```python
from build123d import *

# Parameters (mm, degrees)
SKETCH3_W           = 0.5
SKETCH3_H           = 0.5
BOSS_EXTRUDE1_DEPTH = 10
SKETCH4_W           = 0.5
SKETCH4_H           = 0.5
BOSS_EXTRUDE2_DEPTH = 5
SKETCH5_R           = 0.5
BOSS_EXTRUDE3_DEPTH = 5


with BuildPart() as part:
    # Sketch2 → Revolve1 (revolve)
    with BuildSketch(Plane.XY, mode=Mode.PRIVATE) as revolve1_sk:
        Polygon((0, 0), (2.48, 0), (2.37, 7.9), (0, 7.9), align=None)
    revolve(revolve1_sk.sketch.rotate(Axis((0, 7.9, 0), (0, -1, 0)), 180), axis=Axis((0, 7.9, 0), (0, -1, 0)))

    # Sketch3 → Boss-Extrude1 (add)
    with BuildSketch(Plane.XZ):
        with Locations((-0.625, 0)):
            Rectangle(SKETCH3_W, SKETCH3_H)
        with Locations((-1.875, 0)):
            Rectangle(SKETCH3_W, SKETCH3_H)
        with Locations((0.625, 0)):
            Rectangle(SKETCH3_W, SKETCH3_H)
        with Locations((1.875, 0)):
            Rectangle(SKETCH3_W, SKETCH3_H)
    extrude(amount=BOSS_EXTRUDE1_DEPTH)

    # Sketch4 → Boss-Extrude2 (add)
    with BuildSketch(Plane.XY.offset(-0.25)):
        with Locations((-1.875, -9.75)):
            Rectangle(SKETCH4_W, SKETCH4_H)
        with Locations((-0.625, -9.75)):
            Rectangle(SKETCH4_W, SKETCH4_H)
        with Locations((0.625, -9.75)):
            Rectangle(SKETCH4_W, SKETCH4_H)
        with Locations((1.875, -9.75)):
            Rectangle(SKETCH4_W, SKETCH4_H)
    extrude(amount=-BOSS_EXTRUDE2_DEPTH)

    # Sketch5 → Boss-Extrude3 (add)
    with BuildSketch(Plane.XY.offset(0.25)):
        with Locations(Location((0, -9.75, 0), (0, 0, 210))):
            Circle(SKETCH5_R)
    extrude(amount=BOSS_EXTRUDE3_DEPTH)


solid = part.part
```
Read the model definition and answer for the solid it produces. Units are mm, in the model's axes. A direction names the side the tool comes from. Give positions to 0.01 mm unless a question says otherwise; leave off trailing zeros. Write each loop counter-clockwise with the first axis right and the second up, starting at its lowest first coordinate (ties: lowest second). Pieces come first, ordered by that corner, then holes. Notation, with made-up numbers: (77.5, 80) - (116.5, 80) arc R10 cw to (116.5, 99) - close; hole circle Ø5 at (84.25, -8). An arc over 180 degrees is marked (long way). Write item = value, one per line. Start each with the question number.
Item 1: Each of these flat-tipped pins is pushed along its axis until it touches: P1, Ø1.5, axis at y = -6.5, z = 0.5, coming from the +X side (3 decimals); P2, Ø2, axis at x = 0, y = -0.5, coming from the -Z side; P3, Ø2, axis at x = -1.5, z = -3.5, coming from the -Y side. Where does it stop, or does it pass through?
Item 2: A tool of negligible diameter and unlimited length cuts with its end or side. For faces 5 (the conical face through (-2.31, 4.01, -0.73)), 6 (the flat face through (-0.875, -6, 0)), 7 (the flat face through (-0.375, -6, 0)), 8 (the flat face through (-2.125, -6, 0)), from which of +Z, -Z, +X, -X, +Y, -Y can it reach the whole face along a straight path? Write none if from no direction.
Item 3: Find the intervals of material crossed by probe 1 along Y at (x, z) = (-1.9, -0.5); probe 2 along Y at (x, z) = (-1.25, 1.5); probe 3 along Y at (x, z) = (-0.25, 1.25), in increasing order. Write a range as [from, to].
Item 4: Find section B-B (y = -2.75). Give the vertices of the cut face in (x, z) (3 decimals).
Item 5: Find section A-A (z = -3). Give the vertices of the cut face in (x, y) (3 decimals).
Item 6: The mould has two halves that part along X. Classify faces 1 (the cylindrical face through (-0.338, -10.119, 2.715)), 2 (the flat face through (2.125, -6, 0)), 3 (the flat face through (0.375, -6, 0)), 4 (the flat face through (0.875, -6, 0)): +X half, -X half, draft (parallel to the pull), parting line (faces both ways), or undercut.
Item 7: Find section C-C (z = 3.75). Give the vertices of the cut face in (x, y), then the cut area to 3 significant figures.
Response:
q1.P1 = 2.125
q1.P2 = -2.48
q1.P3 = -10
q2.face_5 = +Y
q2.face_6 = +Z, -Z, -Y
q2.face_7 = -Z, -Y
q2.face_8 = +Z, -Z, -X, -Y
q3.probe_1 = [-10, -9.5], [0, 7.9]
q3.probe_2 = [0, 7.9]
q3.probe_3 = [-10.18, -9.32], [0, 7.9]
q4.outline = (-2.125, -0.25) - (-1.625, -0.25) - (-1.625, 0.25) - (-2.125, 0.25) - close; (-0.875, -0.25) - (-0.375, -0.25) - (-0.375, 0.25) - (-0.875, 0.25) - close; (0.375, -0.25) - (0.875, -0.25) - (0.875, 0.25) - (0.375, 0.25) - close; (1.625, -0.25) - (2.125, -0.25) - (2.125, 0.25) - (1.625, 0.25) - close
q5.outline = (-2.125, -10) - (-1.625, -10) - (-1.625, -9.5) - (-2.125, -9.5) - close; (-0.875, -10) - (-0.375, -10) - (-0.375, -9.5) - (-0.875, -9.5) - close; (0.375, -10) - (0.875, -10) - (0.875, -9.5) - (0.375, -9.5) - close; (1.625, -10) - (2.125, -10) - (2.125, -9.5) - (1.625, -9.5) - close
q6.face_1 = parting line
q6.face_2 = +X half
q6.face_3 = undercut
q6.face_4 = undercut
q7.outline = circle Ø1 at (0, -9.75)
q7.area = 0.785 mm²
